from build123d import *

# Parameters (mm, degrees)
BOSS_1_DEPTH    = 66
CUT_2_DEPTH     = 80
CUT_3_DEPTH     = 80
CUT_4_DEPTH     = 80
CUT_5_DEPTH     = 80
CUT_6_DEPTH     = 62.2
CUT_7_DEPTH     = 62.2
CUT_8_DEPTH     = 62.2
CUT_9_DEPTH     = 62.2
S_CUT10_W       = 52
S_CUT10_H       = 48
POCKET_10_DEPTH = 16.2
S_CUT11_W       = 52
S_CUT11_H       = 60
POCKET_11_DEPTH = 36
S_CUT12_W       = 36
S_CUT12_H       = 48
POCKET_12_DEPTH = 6.1
S_CUT13_W       = 7.2
S_CUT13_H       = 32
POCKET_13_DEPTH = 28
S_HOLE14_R      = 2.5
HOLE_14_DEPTH   = 7.2
S_HOLE15_R      = 2.5
HOLE_15_DEPTH   = 7.2
S_HOLE16_R      = 2.5
HOLE_16_DEPTH   = 7.2
S_HOLE17_R      = 2.5
HOLE_17_DEPTH   = 7.2
S_HOLE18_R      = 1.2
HOLE_18_DEPTH   = 7.2
S_HOLE19_R      = 2.3
HOLE_19_DEPTH   = 2
S_HOLE20_R      = 1.2
HOLE_20_DEPTH   = 7.2
S_HOLE21_R      = 2.3
HOLE_21_DEPTH   = 2


with BuildPart() as part:
    # S_prism1 → Boss_1 (new body)
    with BuildSketch(Plane(origin=(-33, 0, 0), x_dir=(0, 0, -1), z_dir=(1, 0, 0))):
        with BuildLine():
            Line((0, -25.0397), (0, 25.0397))
            ThreePointArc((0, 25.0397), (-0.784802451, 27.419203311), (-2.8311, 28.8651))
            Line((-2.8311, 28.8651), (-32.2859, 37.8651))
            ThreePointArc((-32.2859, 37.8651), (-36.042603994, 38.714700597), (-39.8836, 39))
            Line((-39.8836, 39), (-42, 39))
            ThreePointArc((-42, 39), (-56.1421, 33.1421), (-62, 19))
            Line((-62, 19), (-62, -19))
            ThreePointArc((-62, -19), (-56.1421, -33.1421), (-42, -39))
            Line((-42, -39), (-39.8836, -39))
            ThreePointArc((-39.8836, -39), (-36.042603994, -38.714700597), (-32.2859, -37.8651))
            Line((-32.2859, -37.8651), (-2.8311, -28.8651))
            ThreePointArc((-2.8311, -28.8651), (-0.784802451, -27.419203311), (0, -25.0397))
        make_face()
    extrude(amount=BOSS_1_DEPTH)

    # S_pcut2 → Cut_2 (cut)
    with BuildSketch(Plane(origin=(0, -40, 0), x_dir=(1, 0, 0), z_dir=(0, 1, 0))):
        with BuildLine():
            Line((33.6, -62.6), (11, -62.6))
            Line((11, -62.6), (11, -62))
            ThreePointArc((11, -62), (26.5563, -55.5563), (33, -40))
            Line((33, -40), (33.6, -40))
            Line((33.6, -40), (33.6, -62.6))
        make_face()
    extrude(amount=CUT_2_DEPTH, mode=Mode.SUBTRACT)

    # S_pcut3 → Cut_3 (cut)
    with BuildSketch(Plane(origin=(0, -40, 0), x_dir=(1, 0, 0), z_dir=(0, 1, 0))):
        with BuildLine():
            Line((-33.6, -62.6), (-11, -62.6))
            Line((-11, -62.6), (-11, -62))
            ThreePointArc((-11, -62), (-26.5563, -55.5563), (-33, -40))
            Line((-33, -40), (-33.6, -40))
            Line((-33.6, -40), (-33.6, -62.6))
        make_face()
    extrude(amount=CUT_3_DEPTH, mode=Mode.SUBTRACT)

    # S_pcut4 → Cut_4 (cut)
    with BuildSketch(Plane(origin=(0, -40, 0), x_dir=(1, 0, 0), z_dir=(0, 1, 0))):
        with BuildLine():
            Line((33.6, 0.6), (28, 0.6))
            Line((28, 0.6), (28, 0))
            ThreePointArc((28, 0), (31.5355, -1.4645), (33, -5))
            Line((33, -5), (33.6, -5))
            Line((33.6, -5), (33.6, 0.6))
        make_face()
    extrude(amount=CUT_4_DEPTH, mode=Mode.SUBTRACT)

    # S_pcut5 → Cut_5 (cut)
    with BuildSketch(Plane(origin=(0, -40, 0), x_dir=(1, 0, 0), z_dir=(0, 1, 0))):
        with BuildLine():
            Line((-33.6, 0.6), (-28, 0.6))
            Line((-28, 0.6), (-28, 0))
            ThreePointArc((-28, 0), (-31.5355, -1.4645), (-33, -5))
            Line((-33, -5), (-33.6, -5))
            Line((-33.6, -5), (-33.6, 0.6))
        make_face()
    extrude(amount=CUT_5_DEPTH, mode=Mode.SUBTRACT)

    # S_pcut6 → Cut_6 (cut)
    with BuildSketch(Plane.XY.offset(-0.1)):
        with BuildLine():
            Line((33.6, 39.6), (13, 39.6))
            Line((13, 39.6), (13, 39))
            ThreePointArc((13, 39), (27.1421, 33.1421), (33, 19))
            Line((33, 19), (33.6, 19))
            Line((33.6, 19), (33.6, 39.6))
        make_face()
    extrude(amount=CUT_6_DEPTH, mode=Mode.SUBTRACT)

    # S_pcut7 → Cut_7 (cut)
    with BuildSketch(Plane.XY.offset(-0.1)):
        with BuildLine():
            Line((33.6, -39.6), (13, -39.6))
            Line((13, -39.6), (13, -39))
            ThreePointArc((13, -39), (27.1421, -33.1421), (33, -19))
            Line((33, -19), (33.6, -19))
            Line((33.6, -19), (33.6, -39.6))
        make_face()
    extrude(amount=CUT_7_DEPTH, mode=Mode.SUBTRACT)

    # S_pcut8 → Cut_8 (cut)
    with BuildSketch(Plane.XY.offset(-0.1)):
        with BuildLine():
            Line((-33.6, 39.6), (-13, 39.6))
            Line((-13, 39.6), (-13, 39))
            ThreePointArc((-13, 39), (-27.1421, 33.1421), (-33, 19))
            Line((-33, 19), (-33.6, 19))
            Line((-33.6, 19), (-33.6, 39.6))
        make_face()
    extrude(amount=CUT_8_DEPTH, mode=Mode.SUBTRACT)

    # S_pcut9 → Cut_9 (cut)
    with BuildSketch(Plane.XY.offset(-0.1)):
        with BuildLine():
            Line((-33.6, -39.6), (-13, -39.6))
            Line((-13, -39.6), (-13, -39))
            ThreePointArc((-13, -39), (-27.1421, -33.1421), (-33, -19))
            Line((-33, -19), (-33.6, -19))
            Line((-33.6, -19), (-33.6, -39.6))
        make_face()
    extrude(amount=CUT_9_DEPTH, mode=Mode.SUBTRACT)

    # S_cut10 → Pocket_10 (cut)
    with BuildSketch(Plane.XY.offset(-0.1)):
        Rectangle(S_CUT10_W, S_CUT10_H)
    extrude(amount=POCKET_10_DEPTH, mode=Mode.SUBTRACT)

    # S_cut11 → Pocket_11 (cut)
    with BuildSketch(Plane.XY.offset(16)):
        Rectangle(S_CUT11_W, S_CUT11_H)
    extrude(amount=POCKET_11_DEPTH, mode=Mode.SUBTRACT)

    # S_cut12 → Pocket_12 (cut)
    with BuildSketch(Plane.XY.offset(51.9)):
        Rectangle(S_CUT12_W, S_CUT12_H)
    extrude(amount=POCKET_12_DEPTH, mode=Mode.SUBTRACT)

    # S_cut13 → Pocket_13 (cut)
    with BuildSketch(Plane.XY.offset(16)):
        with Locations((-29.5, 0)):
            Rectangle(S_CUT13_W, S_CUT13_H)
    extrude(amount=POCKET_13_DEPTH, mode=Mode.SUBTRACT)

    # S_hole14 → Hole_14 (cut)
    with BuildSketch(Plane(origin=(25.9, 0, 0), x_dir=(0, 0, -1), z_dir=(1, 0, 0))):
        with Locations(Location((-49, 0, 0), (0, 0, 180))):
            Circle(S_HOLE14_R)
    extrude(amount=HOLE_14_DEPTH, mode=Mode.SUBTRACT)

    # S_hole15 → Hole_15 (cut)
    with BuildSketch(Plane(origin=(25.9, 0, 0), x_dir=(0, 0, -1), z_dir=(1, 0, 0))):
        with Locations(Location((-42, 7, 0), (0, 0, 180))):
            Circle(S_HOLE15_R)
    extrude(amount=HOLE_15_DEPTH, mode=Mode.SUBTRACT)

    # S_hole16 → Hole_16 (cut)
    with BuildSketch(Plane(origin=(25.9, 0, 0), x_dir=(0, 0, -1), z_dir=(1, 0, 0))):
        with Locations(Location((-42, -7, 0), (0, 0, 180))):
            Circle(S_HOLE16_R)
    extrude(amount=HOLE_16_DEPTH, mode=Mode.SUBTRACT)

    # S_hole17 → Hole_17 (cut)
    with BuildSketch(Plane(origin=(25.9, 0, 0), x_dir=(0, 0, -1), z_dir=(1, 0, 0))):
        with Locations(Location((-35, 0, 0), (0, 0, 180))):
            Circle(S_HOLE17_R)
    extrude(amount=HOLE_17_DEPTH, mode=Mode.SUBTRACT)

    # S_hole18 → Hole_18 (cut)
    with BuildSketch(Plane(origin=(-33.1, 0, 0), x_dir=(0, 0, -1), z_dir=(1, 0, 0))):
        with Locations((-8, -10)):
            Circle(S_HOLE18_R)
    extrude(amount=HOLE_18_DEPTH, mode=Mode.SUBTRACT)

    # S_hole19 → Hole_19 (cut)
    with BuildSketch(Plane(origin=(-33.1, 0, 0), x_dir=(0, 0, -1), z_dir=(1, 0, 0))):
        with Locations((-8, -10)):
            Circle(S_HOLE19_R)
    extrude(amount=HOLE_19_DEPTH, mode=Mode.SUBTRACT)

    # S_hole20 → Hole_20 (cut)
    with BuildSketch(Plane(origin=(-33.1, 0, 0), x_dir=(0, 0, -1), z_dir=(1, 0, 0))):
        with Locations((-8, 10)):
            Circle(S_HOLE20_R)
    extrude(amount=HOLE_20_DEPTH, mode=Mode.SUBTRACT)

    # S_hole21 → Hole_21 (cut)
    with BuildSketch(Plane(origin=(-33.1, 0, 0), x_dir=(0, 0, -1), z_dir=(1, 0, 0))):
        with Locations((-8, 10)):
            Circle(S_HOLE21_R)
    extrude(amount=HOLE_21_DEPTH, mode=Mode.SUBTRACT)


solid = part.part
Model file for the job. Use its own axes, mm. A direction names the side the tool comes from. Give positions to 0.01 mm unless a question says otherwise; leave off trailing zeros. Loops run counter-clockwise (first coordinate to the right, second up) from the corner with the lowest first, then second, coordinate; pieces in that order, holes last.
Item 1: Slice it at B-B (y = -26). Write the cut outline in (x, z).
Check values:
outline: (-31.73, 1.68) arc R5 ccw to (-29.08, 0.12) - (29.08, 0.12) arc R5 ccw to (31.73, 1.68) - (31.73, 47.35) arc R22 ccw to (18.35, 60.73) - (-18.35, 60.73) arc R22 ccw to (-31.73, 47.35) - close; hole (-26, 16) - (26, 16) - (26, 52) - (-26, 52) - close
Item 2: Drill centre lines: line 1 along Y through (x, z) = (31, 42); line 2 along Z through (x, y) = (-28.2, -10); line 3 along Y through (x, z) = (18, 40). Where is each one in solid material? Low to high.
Check values:
line 1: y = -27.72 to -9.5, -4.5 to 4.5, 9.5 to 27.72
line 2: z = 0 to 6.8, 9.2 to 16, 44 to 53.72
line 3: y = -38.36 to -30, 30 to 38.36
Item 3: Slice it at A-A (z = 35). Write the cut outline in (x, y), plus the area to 3 significant figures.
Check values:
outline: (-33, -19) arc R20 ccw to (-17.28, -38.54) - (17.28, -38.54) arc R20 ccw to (33, -19) - (33, -2.5) - (26, -2.5) - (26, -30) - (-26, -30) - (-26, -16) - (-33, -16) - close; (-33, 16) - (-26, 16) - (-26, 30) - (26, 30) - (26, 2.5) - (33, 2.5) - (33, 19) arc R20 ccw to (17.28, 38.54) - (-17.28, 38.54) arc R20 ccw to (-33, 19) - close
area: 1,400 mm2
Item 4: Slice it at D-D (z = 27). Write the cut outline in (x, y).
Check values:
outline: (-33, -19) arc R20 ccw to (-23.12, -36.25) - (23.12, -36.25) arc R20 ccw to (33, -19) - (33, 19) arc R20 ccw to (23.12, 36.25) - (-23.12, 36.25) arc R20 ccw to (-33, 19) - (-33, 16) - (-26, 16) - (-26, 30) - (26, 30) - (26, -30) - (-26, -30) - (-26, -16) - (-33, -16) - close
Item 5: Drop flat-ended pins along their axis: P1, Ø2, axis at x = -11, z = 24, coming from the -Y side; P2, Ø1, axis at x = -24.5, y = -25, coming from the +Z side; P3, Ø8, axis at x = 9.5, z = 9.5, coming from the +Y side (3 decimals); P4, Ø11, axis at x = 8.5, z = 35.5, coming from the -Y side. Give the stop position or say it passes through.
Check values:
P1: stops at y = -35.64
P2: stops at z = 57.75
P3: stops at y = 32.125
P4: stops at y = -39
Item 6: Which spindle directions (+Z, -Z, +X, -X, +Y, -Y) get a long thin tool onto all of the face, cutting with end or side? Do faces 1 (the face through (-26, 0, 14)), 2 (the face through (29.5, -5.5, 40)), 3 (the face through (-0.372, 33.297, 55.986)), 4 (the face through (-30, 16, 30)), 5 (the face through (-0.426, -33.428, 17.765)). Say none if no direction does.
Check values:
face 1: none
face 2: +X
face 3: +Z, +X, -X, +Y
face 4: -X
face 5: -Z, +X, -X, -Y
Item 7: Mould opens along Y. For faces 6 (the face through (-28.59, 8.83, 8.26)), 7 (the face through (-0.43, 33.3, 17.35)), 8 (the face through (-31, 0, 1)) say: +Y half, -Y half, draft (parallel to the pull), parting line (faces both ways), or undercut.
Check values:
face 6: undercut
face 7: +Y half
face 8: draft
Item 8: Slice it at C-C (x = -8). Write the cut outline in (y, z), plus the area to 3 significant figures.
Check values:
outline: (-39, 39.88) arc R26 ccw to (-37.87, 32.29) - (-28.87, 2.83) arc R4 ccw to (-25.04, 0) - (-24, 0) - (-24, 16) - (-30, 16) - (-30, 52) - (-24, 52) - (-24, 58) - (24, 58) - (24, 52) - (30, 52) - (30, 16) - (24, 16) - (24, 0) - (25.04, 0) arc R4 ccw to (28.87, 2.83) - (37.87, 32.29) arc R26 ccw to (39, 39.88) - (39, 42) arc R20 ccw to (19, 62) - (-19, 62) arc R20 ccw to (-39, 42) - close
area: 1,050 mm2
